Source: three-view drawing plus pictorial views. Frame: mm from the lowest corner of the part. A direction names the side the tool comes from. Coordinates: 2 decimals unless noted, no trailing zeros. Loops run counter-clockwise (first coordinate to the right, second up) from the corner with the lowest first, then second, coordinate; pieces in that order, holes last. Notation, with made-up numbers: M 30.25,54.25 L 37.25,54.25 A30 ccw 37.25,79.25 Z; hole C 80,18 d2. An arc over 180 degrees is marked long. Use a Markdown table: item, result. Add a question column.
1. Section D-D on x = 5.25. Output: boundary loops of the cut face in (y, z) (3 decimals).
2. Draft query along Z for the marked faces 1, 2 and 3. Return one class per face: +Z half, -Z half, draft (parallel to the pull), parting line (faces both ways), or undercut.
3. Section C-C on z = 22.5. Output: boundary loops of the cut face in (x, y).
4. Set-up query: the marked faces 4 and 5. Return all of +Z, -Z, +X, -X, +Y, -Y with unobstructed straight access to the full face (end or side cutting, diameter ignored); none if empty.
5. Section A-A on y = 28.4. Output: boundary loops of the cut face in (x, z).
6. Section B-B on z = 28.4. Output: boundary loops of the cut face in (x, y), then the cut area to 3 significant figures.
7. Line query: L1, parallel to Y at x = 13, z = 28.4; L2, parallel to X at y = 4, z = 31; L3, parallel to Y at x = 12.5, z = 22. Output: solid intervals per line, ascending. Write a range as [from, to].
8. Pin query (flat end, axial travel): pin 1 (10 mm diameter, centred on x = 3.5, z = 40.5, fed in from -Y); pin 2 (6 mm diameter, centred on y = 40.28, z = 48.97, fed in from +X); pin 3 (3 mm diameter, centred on y = 40.28, z = 7.83, fed in from -X); pin 4 (10 mm diameter, centred on y = 23, z = 30.5, fed in from -X). Return the tip coordinate at first contact, or that it passes through.
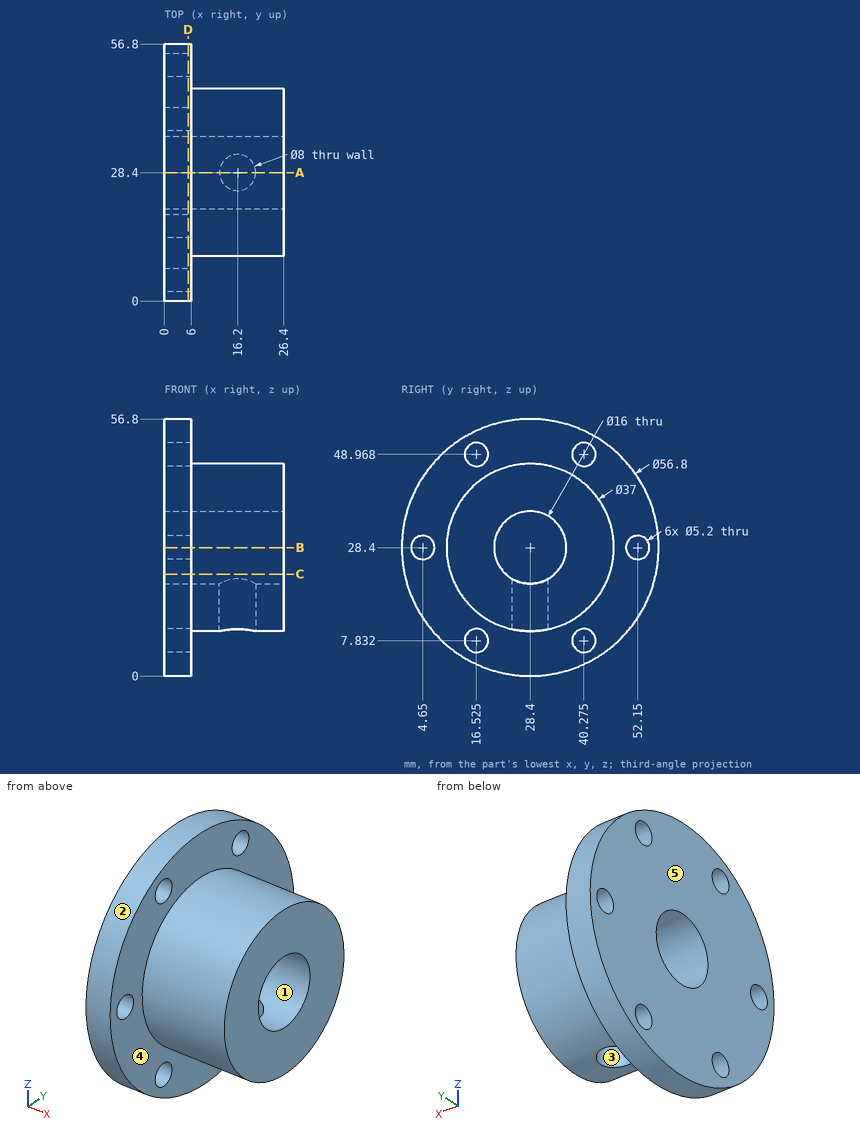
Answers below:
| question | item | result |
|---|---|---|
| 1 | outline | C 28.4,28.4 d56.8; hole C 4.65,28.4 d5.2; hole C 16.525,7.832 d5.2; hole C 16.525,48.968 d5.2; hole C 28.4,28.4 d16; hole C 40.275,7.832 d5.2; hole C 40.275,48.968 d5.2; hole C 52.15,28.4 d5.2 |
| 2 | face 1 | undercut |
| 2 | face 2 | parting line |
| 2 | face 3 | draft |
| 3 | outline | M 0,0.62 L 6,0.62 L 6,10.87 L 26.4,10.87 L 26.4,23 L 0,23 Z; M 0,33.8 L 26.4,33.8 L 26.4,45.93 L 6,45.93 L 6,56.18 L 0,56.18 Z |
| 4 | face 4 | +X |
| 4 | face 5 | +Z, -Z, -X, +Y, -Y |
| 5 | outline | M 0,0 L 6,0 L 6,9.9 L 12.2,9.9 L 12.2,20.4 L 0,20.4 Z; M 0,36.4 L 26.4,36.4 L 26.4,46.9 L 6,46.9 L 6,56.8 L 0,56.8 Z; M 20.2,9.9 L 26.4,9.9 L 26.4,20.4 L 20.2,20.4 Z |
| 6 | outline | M 0,0 L 6,0 L 6,2.05 L 0,2.05 Z; M 0,7.25 L 6,7.25 L 6,9.9 L 26.4,9.9 L 26.4,20.4 L 0,20.4 Z; M 0,36.4 L 26.4,36.4 L 26.4,46.9 L 6,46.9 L 6,49.55 L 0,49.55 Z; M 0,54.75 L 6,54.75 L 6,56.8 L 0,56.8 Z |
| 6 | area | 611 mm² |
| 7 | L1 | y = [9.9, 20.4], [36.4, 46.9] |
| 7 | L2 | x = [0, 6] |
| 7 | L3 | y = [11.04, 23.6], [33.2, 45.76] |
| 8 | pin 1 | stops at y = 0.9 |
| 8 | pin 2 | stops at x = 6 |
| 8 | pin 3 | passes through |
| 8 | pin 4 | stops at x = 0 |
